Study the drawing (mm; zero at the part's minimum x, y, z) and answer. A direction names the side the tool comes from. Coordinates: 2 decimals unless noted, no trailing zeros. Loops run counter-clockwise (first coordinate to the right, second up) from the corner with the lowest first, then second, coordinate; pieces in that order, holes last. Notation, with made-up numbers: (25, -6) - (74, -6) arc R36 cw to (74, 32) - close; hole circle Ø10 at (-1.5, 67.5). An arc over 180 degrees is marked (long way). Use one line per item in the form item = value.
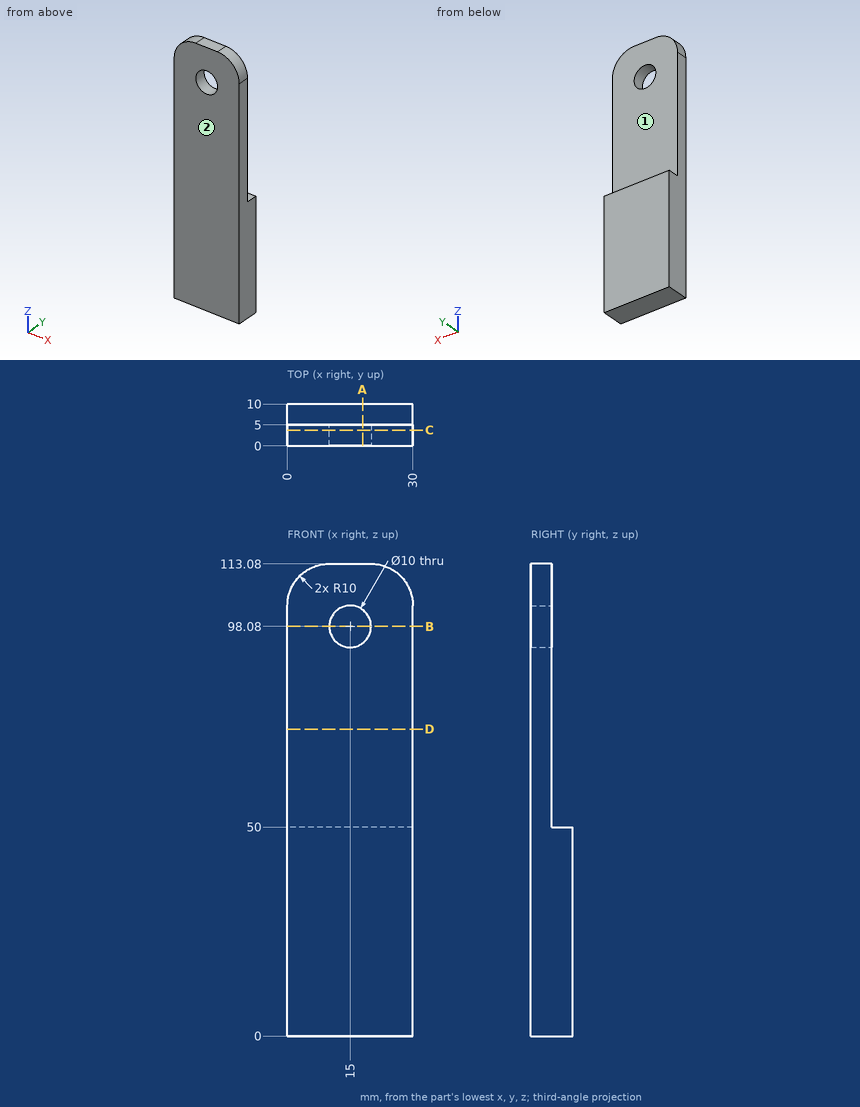
Item 1: Which of the six approach directions +Z, -Z, +X, -X, +Y, -Y give full straight-line access (tool end or side, diameter ignored) to the marked faces 1 and 2?
Results below:
face_1 = +Z, +X, -X, +Y
face_2 = +Z, -Z, +X, -X, -Y
Item 2: The part is cut by section C-C on y = 3.75. Give the vertices of the cut face in (x, z), plus the area to 3 significant figures.
Results below:
outline = (0, 0) - (30, 0) - (30, 103.08) arc R10 ccw to (20, 113.08) - (10, 113.08) arc R10 ccw to (0, 103.08) - close; hole circle Ø10 at (15, 98.08)
area = 3,270 mm²
Item 3: The part is cut by section A-A on x = 18. Give the vertices of the cut face in (y, z), plus the area to 3 significant figures.
Results below:
outline = (0, 0) - (10, 0) - (10, 50) - (5, 50) - (5, 94.08) - (0, 94.08) - close; (0, 102.08) - (5, 102.08) - (5, 113.08) - (0, 113.08) - close
area = 775 mm²
Item 4: Find the intervals of material crossed by L1, parallel to Z at x = 15, y = 2.25; L2, parallel to Y at x = 3, z = 76; L3, parallel to Z at x = 8.5, y = 9, in increasing order.
Results below:
L1 = 0 to 93.08, 103.08 to 113.08
L2 = 0 to 5
L3 = 0 to 50
Item 5: Each of these flat-tipped pins is pushed along its axis until it touches: P1, Ø15, axis at x = 10, z = 90.5, coming from the +Y side; P2, Ø4, axis at x = 18, y = 8, coming from the +Z side; P3, Ø6, axis at x = 15, z = 98.08, coming from the +Y side. Where does it stop, or does it pass through?
Results below:
P1 = 5
P2 = 50
P3 = through
Item 6: The part is cut by section D-D on z = 73.5. Give the vertices of the cut face in (x, y), plus the area to 3 significant figures.
Results below:
outline = (0, 0) - (30, 0) - (30, 5) - (0, 5) - close
area = 150 mm²
Item 7: The part is cut by section B-B on z = 98.08. Give the vertices of the cut face in (x, y), plus the area to 3 significant figures.
Results below:
outline = (0, 0) - (10, 0) - (10, 5) - (0, 5) - close; (20, 0) - (30, 0) - (30, 5) - (20, 5) - close
area = 100 mm²
